Design review of the part shown in the three views and the two pictorial views. Dimensions are in mm from the part's minimum x, y and z. A direction names the side the tool comes from. Give positions to 0.01 mm unless a question says otherwise; leave off trailing zeros. Write each loop counter-clockwise with the first axis right and the second up, starting at its lowest first coordinate (ties: lowest second). Pieces come first, ordered by that corner, then holes. Notation, with made-up numbers: M -35.5,57 L -6.5,57 A10 cw -6.5,63 Z; hole C -26.5,56 d6. An arc over 180 degrees is marked long. Use one line per item in the form item = value. Start each with the question number.
Q1. Consider section B-B on z = 1.7. Write out the cut boundary in (x, y), and give its area (3 significant figures).
Q2. Tool access review of the marked faces 4, 5, 6, 7 and 8: name each direction out of +Z, -Z, +X, -X, +Y, -Y from which nothing blocks a thin tool from reaching the whole face with its end or side.
Q3. Consider section D-D on x = 7. Write out the cut boundary in (y, z), and give its area (3 significant figures).
Q4. Clearance check with flat-ended pins moving along their axes: pin 1 Ø3.5 at (x, y) = (4.5, 6.5) entering from -Z; pin 2 Ø2 at (y, z) = (2.5, 1.5) entering from -X; pin 3 Ø1.2 at (x, y) = (4.5, 2) entering from +Z. State where each tip first meets the part, or that it passes through.
Q5. For probe 1 along X at (y, z) = (6, 1.85); probe 2 along Y at (x, z) = (3.75, 1.5); probe 3 along Z at (x, y) = (4.25, 10), list the stretches that pass through material, from the lowest coordinate up. Write a range as [from, to].
Q6. Consider section C-C on x = 3.75. Write out the cut boundary in (y, z).
Q7. Mouldability with a two-part tool opening along Z and no side actions: class the marked faces 1, 2 and 3 as released by +Z, released by -Z, zero draft, split by the parting line, or undercut.
Q8. Consider section A-A on y = 6. Write out the cut boundary in (x, z), and give its area (3 significant figures).
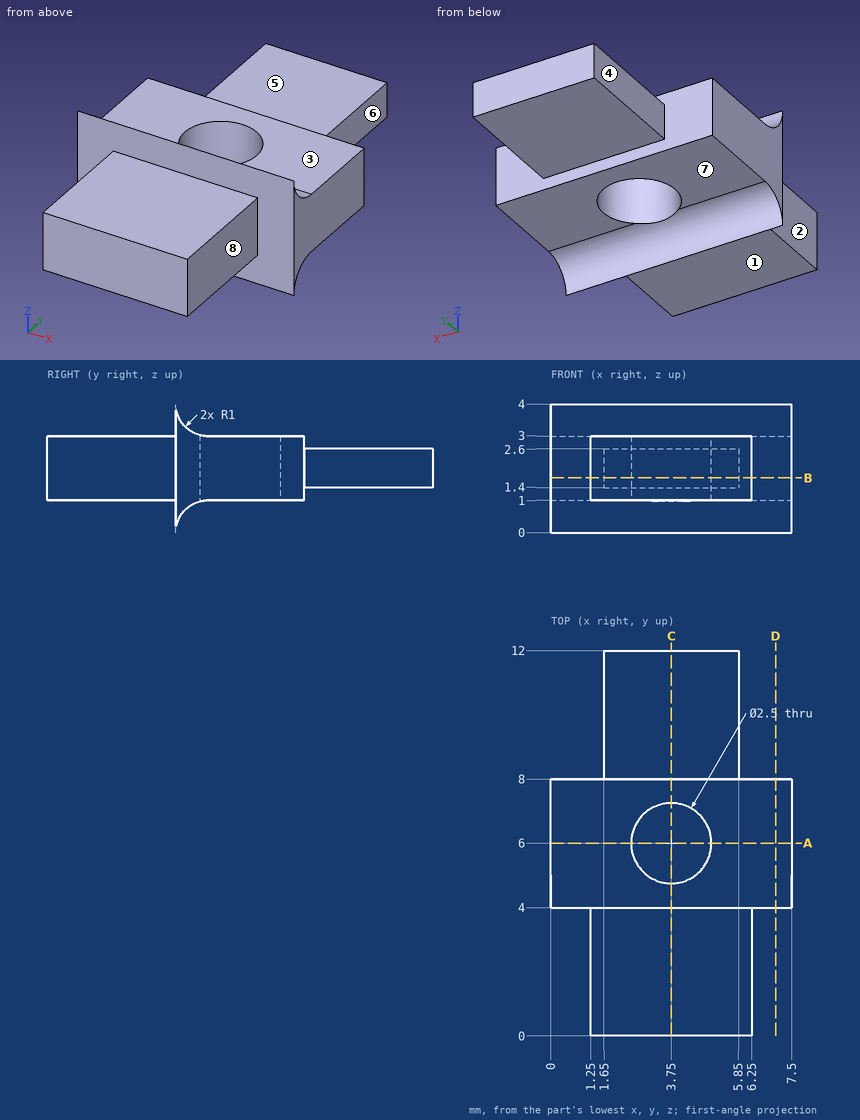
Working result:
q1.outline = M 0,4 L 1.25,4 L 1.25,0 L 6.25,0 L 6.25,4 L 7.5,4 L 7.5,8 L 5.85,8 L 5.85,12 L 1.65,12 L 1.65,8 L 0,8 Z; hole C 3.75,6 d2.5
q1.area = 61.9 mm²
q2.face_4 = +Z, -Z, -X, +Y
q2.face_5 = +Z, +X, -X, +Y
q2.face_6 = +Z, -Z, +X, +Y
q2.face_7 = -Z, +X, -X, +Y
q2.face_8 = +Z, -Z, +X, -Y
q3.outline = M 4,0 A1 cw 5,1 L 8,1 L 8,3 L 5,3 A1 cw 4,4 Z
q3.area = 8.43 mm²
q4.pin_1 = 0.97
q4.pin_2 = 1.25
q4.pin_3 = 3
q5.probe_1 = [0, 2.5], [5, 7.5]
q5.probe_2 = [0, 4.75], [7.25, 12]
q5.probe_3 = [1.4, 2.6]
q6.outline = M 0,1 L 4,1 L 4,0 A1 cw 4.75,0.97 L 4.75,3.03 A1 cw 4,4 L 4,3 L 0,3 Z; M 7.25,1 L 8,1 L 8,1.4 L 12,1.4 L 12,2.6 L 8,2.6 L 8,3 L 7.25,3 Z
q7.face_1 = released by -Z
q7.face_2 = zero draft
q7.face_3 = released by +Z
q8.outline = M 0,1 L 2.5,1 L 2.5,3 L 0,3 Z; M 5,1 L 7.5,1 L 7.5,3 L 5,3 Z
q8.area = 10.0 mm²
